from build123d import *

# Parameters (mm, degrees)
BOSS_EXTRUDE1_DEPTH = 3
SKETCH2_R           = 1.7
CUT_EXTRUDE1_DEPTH  = 43.532340636
BOSS_EXTRUDE2_DEPTH = 1
BOSS_EXTRUDE2_DRAFT = 3
FILLET1_R           = 0.5


with BuildPart() as part:
    # Sketch1 → Boss-Extrude1 (new body)
    with BuildSketch(Plane.XY):
        with BuildLine():
            Line((5, 30), (25, 30))
            ThreePointArc((25, 30), (28.535533906, 28.535533906), (30, 25))
            Line((30, 25), (30, 5))
            ThreePointArc((30, 5), (28.535533906, 1.464466094), (25, 0))
            Line((25, 0), (5, 0))
            ThreePointArc((5, 0), (1.464466094, 1.464466094), (0, 5))
            Line((0, 5), (0, 25))
            ThreePointArc((0, 25), (1.464466094, 28.535533906), (5, 30))
        make_face()
    extrude(amount=BOSS_EXTRUDE1_DEPTH)

    # Sketch2 → Cut-Extrude1 (cut, through all)
    with BuildSketch(Plane.XY.offset(3)):
        with Locations((22.5, 22.5)):
            Circle(SKETCH2_R)
        with Locations((7.5, 7.5)):
            Circle(SKETCH2_R)
        with Locations((7.5, 22.5)):
            Circle(SKETCH2_R)
        with Locations((22.5, 7.5)):
            Circle(SKETCH2_R)
    extrude(amount=-CUT_EXTRUDE1_DEPTH, mode=Mode.SUBTRACT)


with BuildPart() as boss_extrude2_tool:
    # Sketch3 → Boss-Extrude2 (with draft: the straight prism first)
    with BuildSketch(Plane.XY.offset(3)):
        with BuildLine():
            Line((30, 5), (30, 25))
            ThreePointArc((30, 25), (28.535533906, 28.535533906), (25, 30))
            Line((25, 30), (5, 30))
            ThreePointArc((5, 30), (1.464466094, 28.535533906), (0, 25))
            Line((0, 25), (0, 5))
            ThreePointArc((0, 5), (1.464466094, 1.464466094), (5, 0))
            Line((5, 0), (25, 0))
            ThreePointArc((25, 0), (28.535533906, 1.464466094), (30, 5))
        make_face()
        with BuildLine():
            Line((28.5, 25), (28.5, 5))
            ThreePointArc((28.5, 5), (27.474873734, 2.525126266), (25, 1.5))
            Line((25, 1.5), (5, 1.5))
            ThreePointArc((5, 1.5), (2.525126266, 2.525126266), (1.5, 5))
            Line((1.5, 5), (1.5, 25))
            ThreePointArc((1.5, 25), (2.525126266, 27.474873734), (5, 28.5))
            Line((5, 28.5), (25, 28.5))
            ThreePointArc((25, 28.5), (27.474873734, 27.474873734), (28.5, 25))
        make_face(mode=Mode.SUBTRACT)
    extrude(amount=BOSS_EXTRUDE2_DEPTH)
    # Boss-Extrude2: the draft: its side faces are tilted about the plane it starts from
    boss_extrude2_sides = [boss_extrude2_tool.faces().sort_by_distance(p)[0] for p in [
        (15, 0, 3.5),
        (28.535533906, 1.464466094, 3.5),
        (30, 15, 3.5),
        (28.535533906, 28.535533906, 3.5),
        (15, 30, 3.5),
        (1.464466094, 28.535533906, 3.5),
        (0, 15, 3.5),
        (1.464466094, 1.464466094, 3.5),
        (28.5, 15, 3.5),
        (27.474873734, 2.525126266, 3.5),
        (15, 1.5, 3.5),
        (2.525126266, 2.525126266, 3.5),
        (1.5, 15, 3.5),
        (2.525126266, 27.474873734, 3.5),
        (15, 28.5, 3.5),
        (27.474873734, 27.474873734, 3.5),
    ]]
    draft(boss_extrude2_sides, Plane.XY.offset(3), BOSS_EXTRUDE2_DRAFT)


with BuildPart() as part_1:
    add(part.part)

    # Boss-Extrude2: add boss_extrude2_tool
    add(boss_extrude2_tool.part)

    # Fillet1
    fillet1_edges = [part_1.edges().sort_by_distance(p)[0] for p in [
        (28.49847601, 1.50152399, 4),
        (29.947592221, 15, 4),
        (28.49847601, 28.49847601, 4),
        (15, 29.947592221, 4),
        (1.50152399, 28.49847601, 4),
        (0.052407779, 15, 4),
        (1.50152399, 1.50152399, 4),
        (15, 0.052407779, 4),
        (2.48806837, 2.48806837, 4),
        (15, 1.447592221, 4),
        (27.51193163, 2.48806837, 4),
        (28.552407779, 15, 4),
        (27.51193163, 27.51193163, 4),
        (15, 28.552407779, 4),
        (2.48806837, 27.51193163, 4),
        (1.447592221, 15, 4),
    ]]
    fillet(fillet1_edges, radius=FILLET1_R)


solid = part_1.part
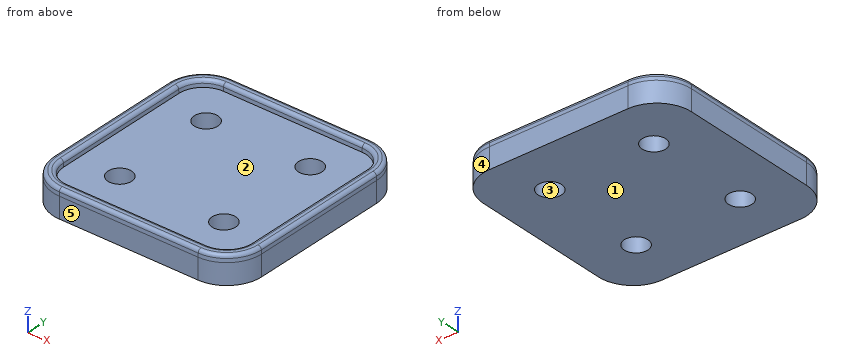
Verification items for the finished model (mm, model axes). Face numbers are marked on the shaded views. A direction names the side the tool comes from. Round coordinates to 2 decimals unless told otherwise and drop trailing zeros. Loops run counter-clockwise (first coordinate to the right, second up) from the corner with the lowest first, then second, coordinate; pieces in that order, holes last. Notation, with made-up numbers: (78, -40) - (116, -40) arc R26 ccw to (116, -6) - close; hole circle Ø11 at (-28, 79). An arc over 180 degrees is marked (long way). Use a Markdown table: item, result. Add a question column.
1. Section check A-A, the plane x = 7.5. Record the boundary of the cut face in (y, z), plus the area to 3 significant figures.
2. Access from +Z, -Z, +X, -X, +Y, -Y to the whole of each face (thin tool, end or side, straight path). Record for the marked faces 1 and 2.
3. Section check C-C, the plane z = 0.95. Record the boundary of the cut face in (x, y), plus the area to 3 significant figures.
4. Gauge pin test, flat ends, axial feed: pin 1 (2 mm diameter, centred on y = 26, z = 1, fed in from +X); pin 2 (1 mm diameter, centred on x = 19.5, y = 10.5, fed in from +Z). Record the tip position at first contact, or that the pin passes through.
5. Release check for a two-part mould opening along X. For the marked faces 3, 4 and 5 record: released by +X, released by -X, zero draft, split by the parting line, or undercut.
6. Section check D-D, the plane y = 18.75. Record the boundary of the cut face in (x, z).
7. Thickness scan on probe 1 along Y at (x, z) = (22.5, 2); probe 2 along X at (y, z) = (8, 1.35); probe 3 along X at (y, z) = (13, 3.1). Record the ranges inside material, lowest first. Write a range as [from, to].
Checks:
| question | item | result |
|---|---|---|
| 1 | outline | (0, 0) - (5.8, 0) - (5.8, 3) - (1.5, 3) - (1.47, 3.53) arc R0.5 ccw to (0.97, 4) - (0.53, 4) arc R0.5 ccw to (0.03, 3.53) - (0, 3) - close; (9.2, 0) - (20.8, 0) - (20.8, 3) - (9.2, 3) - close; (24.2, 0) - (30, 0) - (30, 3) - (29.97, 3.53) arc R0.5 ccw to (29.47, 4) - (29.03, 4) arc R0.5 ccw to (28.53, 3.53) - (28.5, 3) - (24.2, 3) - close |
| 1 | area | 72.3 mm^2 |
| 2 | face 1 | -Z, +X, -X, +Y, -Y |
| 2 | face 2 | +Z |
| 3 | outline | (0, 5) arc R5 ccw to (5, 0) - (25, 0) arc R5 ccw to (30, 5) - (30, 25) arc R5 ccw to (25, 30) - (5, 30) arc R5 ccw to (0, 25) - close; hole circle Ø3.4 at (7.5, 7.5); hole circle Ø3.4 at (7.5, 22.5); hole circle Ø3.4 at (22.5, 7.5); hole circle Ø3.4 at (22.5, 22.5) |
| 3 | area | 842 mm^2 |
| 4 | pin 1 | stops at x = 30 |
| 4 | pin 2 | stops at z = 3 |
| 5 | face 3 | undercut |
| 5 | face 4 | released by +X |
| 5 | face 5 | zero draft |
| 6 | outline | (0, 0) - (30, 0) - (30, 3) - (29.97, 3.53) arc R0.5 ccw to (29.47, 4) - (29.03, 4) arc R0.5 ccw to (28.53, 3.53) - (28.5, 3) - (1.5, 3) - (1.47, 3.53) arc R0.5 ccw to (0.97, 4) - (0.53, 4) arc R0.5 ccw to (0.03, 3.53) - (0, 3) - close |
| 7 | probe 1 | y = [0, 5.8], [9.2, 20.8], [24.2, 30] |
| 7 | probe 2 | x = [0, 5.88], [9.12, 20.88], [24.12, 30] |
| 7 | probe 3 | x = [0.01, 1.49], [28.51, 29.99] |
